Input: part model. Units: mm. Frame: model coordinates. Face numbers are marked on the shaded views. A direction names the side the tool comes from. Round coordinates to 2 decimals unless told otherwise and drop trailing zeros. Loops run counter-clockwise (first coordinate to the right, second up) from the corner with the lowest first, then second, coordinate; pieces in that order, holes last. Notation, with made-up numbers: (-14, -29) -> (40, -29) arc R27 ccw to (40, -12) -> close; hole circle Ø8 at (-27, 64.25). An arc over 180 degrees is marked (long way). Answer as a JSON object with one key per item and string values. Group by question number.
Item 1: Pin query (flat end, axial travel): pin 1 (6 mm diameter, centred on x = 21, y = -10, fed in from +Z); pin 2 (3 mm diameter, centred on y = -21, z = 0, fed in from -X); pin 3 (8 mm diameter, centred on y = 1, z = 29, fed in from +X); pin 4 (1.5 mm diameter, centred on x = 44, y = -42, fed in from +Z). Return the tip coordinate at first contact, or that it passes through.
Item 2: Section query B-B on y = -29. Return loops of the section in (x, z).
Item 3: Material intervals for line 1 (Y direction, x = 22.5, z = 3.5); line 2 (X direction, y = -27.5, z = 0), sorted ascending. Write a range as [from, to].
Item 4: Set-up query: the marked faces 1, 2 and 3. Return all of +Z, -Z, +X, -X, +Y, -Y with unobstructed straight access to the full face (end or side cutting, diameter ignored); none if empty.
Item 5: Section query D-D on y = -0.5. Return loops of the section in (x, z).
Item 6: Section query C-C on x = 35. Return loops of the section in (y, z), and give its area (3 significant figures).
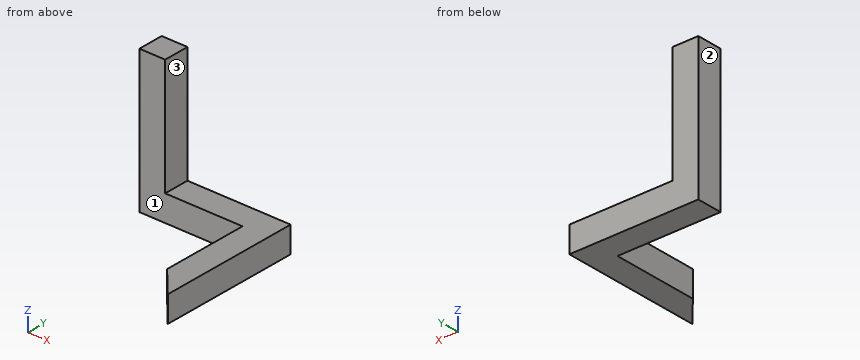
from build123d import *

# Parameters (mm, degrees)
F0_W     = 10
F0_H     = 10
F1_DEPTH = 50
F2_W     = 10
F2_H     = 10
F3_DEPTH = 50
F4_W     = 10
F4_H     = 10
F5_DEPTH = 50
F6_SIZE2 = 9.99999
F6_SIZE  = 11.24999


# Not quite as in the source:
# - a fillet or chamfer is up to 0.001 mm smaller than in the source, because OpenCascade refuses the exact size


with BuildPart() as f1:
    # F0 (on Right) → F1 (new body)
    with BuildSketch(Plane.YZ):
        Rectangle(F0_W, F0_H)
    extrude(amount=F1_DEPTH)

    # F2 (on Top) → F3 (join)
    with BuildSketch(Plane.XY):
        with Locations((5, 0)):
            Rectangle(F2_W, F2_H)
    extrude(amount=F3_DEPTH)

    # F4 (on Front) → F5 (join)
    with BuildSketch(Plane.XZ):
        with Locations((45, 0)):
            Rectangle(F4_W, F4_H)
    extrude(amount=F5_DEPTH)

    # F6 (size 11.25 and 10 in the source; OpenCascade refuses exactly that, so slightly less here)
    f6_edges = [f1.edges().sort_by_distance(p)[0] for p in [
        (40, -50, 0),
    ]]
    f6_side = f1.faces().sort_by_distance((40, -27.5, 0))[0]
    chamfer(f6_edges, length=F6_SIZE, length2=F6_SIZE2, reference=f6_side)


solid = f1.part
Solved:
{
 "1": {"pin 1": "through", "pin 2": "x = 40", "pin 3": "x = 10", "pin 4": "z = 5"},
 "2": {"outline": "(40, -5) -> (50, -5) -> (50, 5) -> (40, 5) -> close"},
 "3": {"line 1": "[-5, 5]", "line 2": "[40, 50]"},
 "4": {"face 1": "+Z, -Z, -X, -Y", "face 2": "+Z, -Z, -X, +Y, -Y", "face 3": "+Z, +X, +Y, -Y"},
 "5": {"outline": "(0, -5) -> (50, -5) -> (50, 5) -> (10, 5) -> (10, 50) -> (0, 50) -> close"},
 "6": {"outline": "(-5, -5) -> (5, -5) -> (5, 5) -> (-5, 5) -> close", "area": "100 mm²"}
}
